```python
from build123d import *

# Parameters (mm, degrees)
BOSS_EXTRUDE1_DEPTH        = 6.35
F_1_4_0_2500_DOWEL_HOLE4_D = 6.35
FILLET1_R                  = 10
FILLET2_R                  = 10
FILLET4_R                  = 5
FILLET5_R                  = 1
FILLET6_R                  = 10


with BuildPart() as part:
    # Sketch1 → Boss-Extrude1 (new body)
    with BuildSketch(Plane(origin=(0, 0, 0), x_dir=(0, 0, -1), z_dir=(1, 0, 0))):
        with BuildLine():
            ThreePointArc((-34.29915969, 59.86223243), (-47.669324906, 54.86223243), (-34.29915969, 49.86223243))
            Line((-34.29915969, 49.86223243), (28.354545267, 49.86223243))
            ThreePointArc((28.354545267, 49.86223243), (34.104710482, 47.24223243), (39.854875697, 49.86223243))
            Line((39.854875697, 49.86223243), (56.104710487, 49.86223243))
            Line((56.104710487, 49.86223243), (58.379362515, 48.80154477))
            add(Edge.make_bspline(
                [(58.379362515, 48.80154477), (58.386228757, 46.363071997), (57.773854653, 43.567008128)],
                knots=[0, 0, 0, 1, 1, 1], degree=2))
            add(Edge.make_bspline(
                [(63.433148606, 46.444925613), (61.354068213, 44.407555536), (57.773854653, 43.567008128)],
                knots=[0.61808465, 0.61808465, 0.61808465, 1, 1, 1], degree=2))
            Line((63.433148606, 46.444925613), (71.973979321, 42.462270844))
            add(Edge.make_bspline(
                [(71.973979321, 42.462270844), (71.980845562, 40.023798071), (71.368471459, 37.227734202)],
                knots=[0, 0, 0, 1, 1, 1], degree=2))
            add(Edge.make_bspline(
                [(77.027765412, 40.105651687), (74.948685018, 38.06828161), (71.368471459, 37.227734202)],
                knots=[0.61808465, 0.61808465, 0.61808465, 1, 1, 1], degree=2))
            Line((77.027765412, 40.105651687), (85.568596126, 36.122996918))
            add(Edge.make_bspline(
                [(85.568596126, 36.122996918), (85.575462368, 33.684524145), (84.963088264, 30.888460276)],
                knots=[0, 0, 0, 1, 1, 1], degree=2))
            add(Edge.make_bspline(
                [(90.622382217, 33.766377761), (88.543301824, 31.729007684), (84.963088264, 30.888460276)],
                knots=[0.61808465, 0.61808465, 0.61808465, 1, 1, 1], degree=2))
            Line((90.622382217, 33.766377761), (99.163212932, 29.783722992))
            add(Edge.make_bspline(
                [(99.163212932, 29.783722992), (98.939072146, 24.65005498), (94.755179462, 18.075155142)],
                knots=[0, 0, 0, 1, 1, 1], degree=2))
            add(Edge.make_bspline(
                [(94.755179462, 18.075155142), (112.208752339, 22.33534385), (106.773416656, 37.268805905)],
                knots=[0.444949083, 0.444949083, 0.444949083, 1.444949083, 1.444949083, 1.444949083], degree=2))
            Line((106.773416656, 37.268805905), (79.825550101, 49.834802449))
            Line((79.825550101, 49.834802449), (58.321657114, 59.86223243))
            Line((58.321657114, 59.86223243), (39.854875697, 59.86223243))
            ThreePointArc((39.854875697, 59.86223243), (34.104710482, 62.48223243), (28.354545266, 59.86223243))
            Line((28.354545266, 59.86223243), (-34.29915969, 59.86223243))
        make_face()
    extrude(amount=BOSS_EXTRUDE1_DEPTH)

    # 1/4 (0.2500) Dowel Hole4 (through all)
    with Locations(Plane(origin=(6.35, 0, 0), x_dir=(0, 0, -1), z_dir=(1, 0, 0))):
        with Locations((-40.049324906, 54.86223243), (34.104710482, 54.86223243)):
            Hole(F_1_4_0_2500_DOWEL_HOLE4_D / 2)

    # Fillet1
    fillet1_edges = [part.edges().sort_by_distance(p)[0] for p in [
        (3.175, 49.86223243, 34.29915969),
        (3.175, 59.86223243, 34.29915969),
    ]]
    fillet(fillet1_edges, radius=FILLET1_R)

    # Fillet2
    fillet2_edges = [part.edges().sort_by_distance(p)[0] for p in [
        (3.175, 49.86223243, -56.104710487),
        (3.175, 59.86223243, -58.321657114),
    ]]
    fillet(fillet2_edges, radius=FILLET2_R)

    # Fillet4
    fillet4_edges = [part.edges().sort_by_distance(p)[0] for p in [
        (3.175, 37.268805905, -106.773416656),
    ]]
    fillet(fillet4_edges, radius=FILLET4_R)

    # Fillet5
    fillet5_edges = [part.edges().sort_by_distance(p)[0] for p in [
        (3.175, 33.766377761, -90.622382217),
        (3.175, 40.105651687, -77.027765412),
        (3.175, 46.444925613, -63.433148606),
        (3.175, 48.80154477, -58.379362515),
        (3.175, 42.462270844, -71.973979321),
        (3.175, 36.122996918, -85.568596126),
        (3.175, 29.783722992, -99.163212932),
    ]]
    fillet(fillet5_edges, radius=FILLET5_R)

    # Fillet6
    fillet6_edges = [part.edges().sort_by_distance(p)[0] for p in [
        (3.175, 49.86223243, -39.854875697),
        (3.175, 49.86223243, -28.354545267),
        (3.175, 59.86223243, -28.354545266),
        (3.175, 59.86223243, -39.854875697),
    ]]
    fillet(fillet6_edges, radius=FILLET6_R)


solid = part.part
```
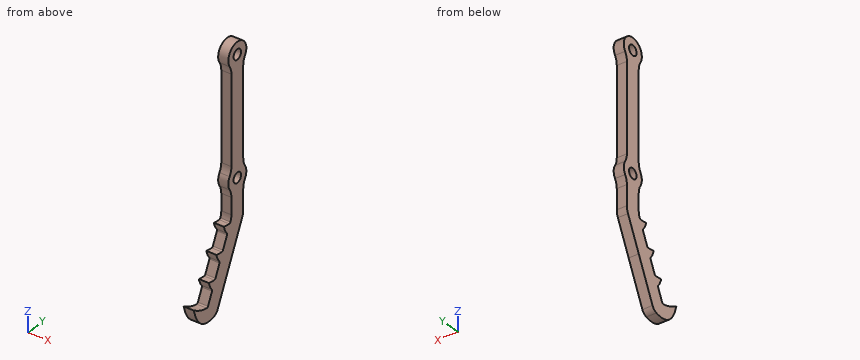
The listing builds one solid part. Answer for the finished solid, in the listing's coordinates (mm). Give positions to 0.01 mm unless a question says otherwise; leave off trailing zeros. Loops run counter-clockwise (first coordinate to the right, second up) from the corner with the lowest first, then second, coordinate; pieces in that order, holes last. Notation, with made-up numbers: M 73.5,17.5 L 132.5,17.5 A19 cw 132.5,38.5 Z; hole C -5,75.25 d5. An arc over 180 degrees is marked long. One line per item, written item: value.
1. Section B-B on x = 2.5 is taken. State how many separate pieces and enclosed holes the cut face has, plus the area to 3 significant figures.
Found:
separate pieces: 1
enclosed holes: 2
area: 1,740 mm^2
2. Section C-C on z = -93 is taken. Determine the outline of the cut face in (x, y).
Found:
outline: M 0,32.66 L 6.35,32.66 L 6.35,43.69 L 0,43.69 Z
3. Section A-A on z = -23 is taken. Determine the outline of the cut face in (x, y), plus the area to 3 significant figures.
Found:
outline: M 0,49.86 L 6.35,49.86 L 6.35,59.86 L 0,59.86 Z
area: 63.5 mm^2
4. Find the intervals of material crossed by probe 1 along Z at (x, y) = (3, 48); probe 2 along Z at (x, y) = (2.75, 56); probe 3 along Z at (x, y) = (4.5, 35), in increasing order.
Found:
probe 1: -83.76 to -58.37, -37.42 to -30.79, 36.74 to 43.36
probe 2: -66.6 to -37.07, -31.14 to 37.09, 43.01 to 47.58
probe 3: -107.48 to -85.54
5. Each of these flat-tipped pins is pushed along its axis until it touches: P1, Ø1, axis at x = 4.5, z = 8.5, coming from the -Y side; P2, Ø1.5, axis at x = 2, z = -41, coming from the +Y side; P3, Ø3, axis at x = 2.5, y = 39.5, coming from the +Z side. Where does it stop, or does it pass through?
Found:
P1: y = 49.86
P2: y = 60.35
P3: z = -71.53
